Design review of the part built by this model. Coordinates are the model's own, in mm. A direction names the side the tool comes from. Coordinates: 2 decimals unless noted, no trailing zeros. Loops run counter-clockwise (first coordinate to the right, second up) from the corner with the lowest first, then second, coordinate; pieces in that order, holes last. Notation, with made-up numbers: (54, 71) - (85, 71) arc R33 cw to (85, 100) - close; hole circle Ø2 at (29.5, 67.5). An arc over 180 degrees is marked (long way). One line per question, with ' | ' between items.
from build123d import *

# Parameters (mm, degrees)
SKETCH1_W                       = 6.35
SKETCH1_H                       = 88.9
BOSS_EXTRUDE1_DEPTH             = 6.35
SKETCH2_W                       = 12.7
SKETCH2_H                       = 6.35
BOSS_EXTRUDE2_DEPTH             = 120.65
SKETCH3_W                       = 12.446
SKETCH3_H                       = 6.35
BOSS_EXTRUDE3_DEPTH             = 120.65
SKETCH1_2_W                     = 6.35
SKETCH1_2_H                     = 88.9
BOSS_EXTRUDE4_DEPTH             = 6.35
SKETCH4_W                       = 6.096
SKETCH4_H                       = 6.35
BOSS_EXTRUDE5_DEPTH             = 120.65
SKETCH5_W                       = 6.096
SKETCH5_H                       = 6.35
BOSS_EXTRUDE6_DEPTH             = 120.65
F_8_32_TAPPED_HOLE1_D           = 3.4544
F_8_32_TAPPED_HOLE1_ON_FACE_2_D = 3.4544
SKETCH7_R                       = 3.175
BOSS_EXTRUDE7_DEPTH             = 12.7
SKETCH8_R                       = 3.175
BOSS_EXTRUDE8_DEPTH             = 12.7
SKETCH9_R                       = 3.175
BOSS_EXTRUDE10_DEPTH            = 12.7
SKETCH10_R                      = 3.175
BOSS_EXTRUDE11_DEPTH            = 12.7
SKETCH12_R                      = 2.38125
CUT_EXTRUDE2_DEPTH              = 127
SKETCH13_R                      = 2.38125
CUT_EXTRUDE3_DEPTH              = 127


with BuildPart() as part:
    # Sketch1 → Boss-Extrude1 (new body)
    with BuildSketch(Plane(origin=(0, 0, 0), x_dir=(1, 0, 0), z_dir=(0, 1, 0))):
        with Locations((-73.025, 0)):
            Rectangle(SKETCH1_W, SKETCH1_H)
    extrude(amount=BOSS_EXTRUDE1_DEPTH)

    # Sketch2 → Boss-Extrude2 (add)
    with BuildSketch(Plane(origin=(-69.85, 0, 0), x_dir=(0, 0, -1), z_dir=(1, 0, 0))):
        with Locations((-38.1, 3.175)):
            Rectangle(SKETCH2_W, SKETCH2_H)
    extrude(amount=BOSS_EXTRUDE2_DEPTH)

    # Sketch3 → Boss-Extrude3 (add)
    with BuildSketch(Plane(origin=(-69.85, 0, 0), x_dir=(0, 0, -1), z_dir=(1, 0, 0))):
        with Locations((38.227, 3.175)):
            Rectangle(SKETCH3_W, SKETCH3_H)
    extrude(amount=BOSS_EXTRUDE3_DEPTH)

    # Sketch1<2> → Boss-Extrude4 (add)
    with BuildSketch(Plane(origin=(0, 0, 0), x_dir=(1, 0, 0), z_dir=(0, 1, 0))):
        with Locations((-73.025, 0)):
            Rectangle(SKETCH1_2_W, SKETCH1_2_H)
    extrude(amount=-BOSS_EXTRUDE4_DEPTH)

    # Sketch4 → Boss-Extrude5 (add)
    with BuildSketch(Plane(origin=(-69.85, 0, 0), x_dir=(0, 0, -1), z_dir=(1, 0, 0))):
        with Locations((-41.402, -3.175)):
            Rectangle(SKETCH4_W, SKETCH4_H)
    extrude(amount=BOSS_EXTRUDE5_DEPTH)

    # Sketch5 → Boss-Extrude6 (add)
    with BuildSketch(Plane(origin=(-69.85, 0, 0), x_dir=(0, 0, -1), z_dir=(1, 0, 0))):
        with Locations((41.402, -3.175)):
            Rectangle(SKETCH5_W, SKETCH5_H)
    extrude(amount=BOSS_EXTRUDE6_DEPTH)

    # #8-32 Tapped Hole1 (through all)
    with Locations(Plane(origin=(45.72, -3.175, -44.45), x_dir=(-1, 0, 0), z_dir=(0, 0, -1))):
        with Locations((0, 0), (38.1, 0)):
            Hole(F_8_32_TAPPED_HOLE1_D / 2)

    # #8-32 Tapped Hole1 on face 2 (through all)
    with Locations(Plane(origin=(45.72, -3.175, 44.45), x_dir=(1, 0, 0), z_dir=(0, 0, 1))):
        with Locations((0, 0), (-38.1, 0)):
            Hole(F_8_32_TAPPED_HOLE1_ON_FACE_2_D / 2)

    # Sketch7 → Boss-Extrude7 (add)
    with BuildSketch(Plane(origin=(-14.456865446, 0, 44.45), x_dir=(1, 0, 0), z_dir=(0, 0, 1))):
        with Locations(Location((27.94, 0, 0), (0, 0, 180))):
            Circle(SKETCH7_R)
    extrude(amount=BOSS_EXTRUDE7_DEPTH)

    # Sketch8 → Boss-Extrude8 (add)
    with BuildSketch(Plane.XY.offset(44.45)):
        with Locations(Location((-38.12905493, 0, 0), (0, 0, 180))):
            Circle(SKETCH8_R)
    extrude(amount=BOSS_EXTRUDE8_DEPTH)

    # Sketch9 → Boss-Extrude10 (add)
    with BuildSketch(Plane(origin=(0, 0, -44.45), x_dir=(-1, 0, 0), z_dir=(0, 0, -1))):
        with Locations(Location((38.1, 0, 0), (0, 0, 180))):
            Circle(SKETCH9_R)
    extrude(amount=BOSS_EXTRUDE10_DEPTH)

    # Sketch10 → Boss-Extrude11 (add)
    with BuildSketch(Plane(origin=(0, 0, -44.45), x_dir=(-1, 0, 0), z_dir=(0, 0, -1))):
        with Locations(Location((-13.97, 0, 0), (0, 0, 180))):
            Circle(SKETCH10_R)
    extrude(amount=BOSS_EXTRUDE11_DEPTH)

    # Sketch12 → Cut-Extrude2 (cut)
    with BuildSketch(Plane(origin=(17.145, 0, 0), x_dir=(0, 0, -1), z_dir=(1, 0, 0))):
        with Locations((50.8, -3.048)):
            Circle(SKETCH12_R)
    extrude(amount=-CUT_EXTRUDE2_DEPTH, mode=Mode.SUBTRACT)

    # Sketch13 → Cut-Extrude3 (cut)
    with BuildSketch(Plane(origin=(17.145, 0, 0), x_dir=(0, 0, -1), z_dir=(1, 0, 0))):
        with Locations((-50.8, -3.175)):
            Circle(SKETCH13_R)
    extrude(amount=-CUT_EXTRUDE3_DEPTH, mode=Mode.SUBTRACT)


solid = part.part
Q1. Draft analysis for pull direction X (two halves, no side actions). For faces 5 (the cylindrical face through (44, -3, 41)), 6 (the cylindrical face through (-38.086, -0.794, 50.748)), 7 (the flat face through (-76.2, 0, 1)), 8 (the flat face through (-14, 0, -44.45)), state which applies: +X half, -X half, draft (parallel to the pull), parting line (faces both ways), or undercut.
Returned:
face 5: undercut | face 6: draft | face 7: -X half | face 8: undercut
Q2. Take a section at B-B (x = 45.72). Give the boundary of the cut face in (y, z).
Returned:
outline: (-6.35, -44.45) - (-4.9, -44.45) - (-4.9, -38.35) - (-6.35, -38.35) - close; (-6.35, 38.35) - (-4.9, 38.35) - (-4.9, 44.45) - (-6.35, 44.45) - close; (-1.45, -44.45) - (6.35, -44.45) - (6.35, -32) - (0, -32) - (0, -38.35) - (-1.45, -38.35) - close; (-1.45, 38.35) - (0, 38.35) - (0, 31.75) - (6.35, 31.75) - (6.35, 44.45) - (-1.45, 44.45) - close
Q3. Take a section at A-A (x = -47). Give the boundary of the cut face in (y, z).
Returned:
outline: (-6.35, -44.45) - (6.35, -44.45) - (6.35, -32) - (0, -32) - (0, -38.35) - (-6.35, -38.35) - close; (-6.35, 38.35) - (0, 38.35) - (0, 31.75) - (6.35, 31.75) - (6.35, 44.45) - (-6.35, 44.45) - close
Q4. For pin 1 (7 mm diameter, centred on x = -9.5, y = -2, fed in from +Z); pin 2 (5 mm diameter, centred on x = -30, y = 4.5, fed in from -Z); pin 3 (4 mm diameter, centred on x = 7.62, y = -3.175, fed in from -Z), all flat-tipped, find the tip position at first contact; note any pin that passes through.
Returned:
pin 1: stops at z = 44.45 | pin 2: stops at z = -44.45 | pin 3: stops at z = -44.45
Q5. To check wall thickness, follow line 1 along Z through (x, y) = (17.5, -4.25); line 2 along Y through (x, z) = (7.62, 42.5); line 3 along Z through (x, y) = (24, 1.5). State the ranges of each line that lie inside material, in increasing order.
Returned:
line 1: z = -44.45 to -38.35, 38.35 to 44.45 | line 2: y = -6.35 to -4.9, -1.45 to 6.35 | line 3: z = -44.45 to -32, 31.75 to 44.45
Q6. Take a section at C-C (y = 4.75). Give the boundary of the cut face in (x, z), plus the area to 3 significant figures.
Returned:
outline: (-76.2, -44.45) - (50.8, -44.45) - (50.8, -32) - (-69.85, -32) - (-69.85, 31.75) - (50.8, 31.75) - (50.8, 44.45) - (-76.2, 44.45) - close | area: 3,600 mm²
Q7. Tool access review of faces 1 (the cylindrical face through (13.28, 3.1, -50.71)), 2 (the cylindrical face through (-37.44, 3.1, 50.71)), 3 (the flat face through (-10, 3, -32.004)), 4 (the flat face through (-10, -3, 38.354)): name each direction out of +Z, -Z, +X, -X, +Y, -Y from which nothing blocks a thin tool from reaching the whole face with its end or side.
Returned:
face 1: -Z | face 2: +Z | face 3: +X, +Y, -Y | face 4: +X, -Y
Q8. Take a section at D-D (z = -50.8). Give the boundary of the cut face in (x, y) (3 decimals), plus the area to 3 significant figures.
Returned:
outline: (-41.204, -0.667) - (-34.996, -0.667) arc R3.175 ccw (long way) to start; (10.866, -0.667) - (17.074, -0.667) arc R3.175 ccw (long way) to start | area: 40.1 mm²
